from build123d import *

# Parameters (mm, degrees)
BOSS_EXTRUDE1_DEPTH = 3


with BuildPart() as part:
    # Sketch1 → Boss-Extrude1 (new body)
    with BuildSketch(Plane(origin=(0, 0, 0), x_dir=(1, 0, 0), z_dir=(0, 1, 0))):
        with BuildLine():
            Line((-3, -24), (-3, -30))
            Line((-3, -30), (-10, -30))
            Line((-10, -30), (-10, -5))
            Line((-10, -5), (-13, -5))
            Line((-13, -5), (-13, 5))
            Line((-13, 5), (-10, 5))
            Line((-10, 5), (-10, 30))
            Line((-10, 30), (-5, 30))
            Line((-5, 30), (-5, 27))
            Line((-5, 27), (5, 27))
            Line((5, 27), (5, 30))
            Line((5, 30), (10, 30))
            Line((10, 30), (10, -18))
            Line((10, -18), (3, -18))
            ThreePointArc((3, -18), (-1.242640687, -19.757359313), (-3, -24))
        make_face()
    extrude(amount=BOSS_EXTRUDE1_DEPTH)


solid = part.part
The listing builds one solid part. Answer for the finished solid, in the listing's coordinates (mm). A direction names the side the tool comes from. Coordinates: 2 decimals unless noted, no trailing zeros. Order: outer loops, then holes, each group sorted by start corner. A loop starts at its lowest first (then second) coordinate and runs counter-clockwise, first axis right, second up.
Q1. Consider line 1 (X direction, y = 1.8, z = 11.5); line 2 (X direction, y = 1.2, z = 24); line 3 (Z direction, x = 5.25, y = 2.3). Determine where each line is inside the solid, lowest interval first.
Q2. For a pull along X with two mould halves and no side action, classify faces 5 (the face through (-3, 1, 27)), 6 (the face through (-12, 1, -5)), 7 (the face through (-10, 1, -17)), 8 (the face through (0, 1, -27)) as pulls with the +X half, pulls with the -X half, needs draft (parallel to the pull), parting line crosses it, or undercut.
Q3. A cutting plane is placed at B-B, the plane x = -11.5. Write down the section's boundary in (y, z).
Q4. Given P1, Ø1.5, axis at x = 8, y = 2, coming from the +Z side; P2, Ø0.9, axis at y = 1, z = 16, coming from the -X side; P3, Ø0.9, axis at x = 1, y = 1.5, coming from the -Z side, each flat-ended and moving along its own axis, determine where each tip first touches the part or whether it passes through.
Q5. A cutting plane is placed at C-C, the plane z = -7.5. Write down the section's boundary in (x, y).
Q6. A cutting plane is placed at A-A, the plane y = 1.65. Write down the section's boundary in (x, z).
Q7. Which of the six approach directions +Z, -Z, +X, -X, +Y, -Y give full straight-line access (tool end or side, diameter ignored) to faces 1 (the face through (7, 1, 18)), 2 (the face through (5, 1, -28)), 3 (the face through (7, 1, -30)), 4 (the face through (-10, 1, 18))?
Answers follow:
1. line 1: x = -10 to 10
1. line 2: x = -10 to -3
1. line 3: z = -30 to 18
2. face 5: pulls with the +X half
2. face 6: needs draft
2. face 7: pulls with the -X half
2. face 8: undercut
3. outline: (0, -5) - (3, -5) - (3, 5) - (0, 5) - close
4. P1: stops at z = 18
4. P2: stops at x = -10
4. P3: stops at z = -27
5. outline: (-10, 0) - (10, 0) - (10, 3) - (-10, 3) - close
6. outline: (-13, -5) - (-10, -5) - (-10, -30) - (-5, -30) - (-5, -27) - (5, -27) - (5, -30) - (10, -30) - (10, 18) - (3, 18) arc R6 cw to (-3, 24) - (-3, 30) - (-10, 30) - (-10, 5) - (-13, 5) - close
7. face 1: +Z, +X, +Y, -Y
7. face 2: -Z, +Y, -Y
7. face 3: -Z, +X, -X, +Y, -Y
7. face 4: +Z, -X, +Y, -Y
